from build123d import *

# Parameters (mm, degrees)
SKETCH1_W           = 30
SKETCH1_H           = 100
BOSS_EXTRUDE1_DEPTH = 5
SKETCH2_W           = 30
SKETCH2_H           = 45
BOSS_EXTRUDE2_DEPTH = 5
SKETCH3_W           = 30
SKETCH3_H           = 5
BOSS_EXTRUDE3_DEPTH = 15
SKETCH4_R           = 2.5
CUT_EXTRUDE1_DEPTH  = 8
SKETCH5_W           = 6
SKETCH5_H           = 5
CUT_EXTRUDE2_DEPTH  = 20


with BuildPart() as part:
    # Sketch1 → Boss-Extrude1 (new body)
    with BuildSketch(Plane.XY):
        with Locations((11.532089338, -8.646905221)):
            Rectangle(SKETCH1_W, SKETCH1_H)
        with BuildLine():
            Line((14.615865264, 31.346811585), (14.448313411, -48.653188415))
            ThreePointArc((14.448313411, -48.653188415), (11.442030217, -51.646905221), (8.448313411, -48.640622026))
            Line((8.448313411, -48.640622026), (8.615865264, 31.359377974))
            ThreePointArc((8.615865264, 31.359377974), (11.622148459, 34.353094779), (14.615865264, 31.346811585))
        make_face(mode=Mode.SUBTRACT)
    extrude(amount=BOSS_EXTRUDE1_DEPTH)

    # Sketch2 → Boss-Extrude2 (add)
    with BuildSketch(Plane(origin=(0, 41.353094779, 0), x_dir=(1, 0, 0), z_dir=(0, 1, 0))):
        with Locations((11.532089338, -2.5)):
            Rectangle(SKETCH2_W, SKETCH2_H)
    extrude(amount=BOSS_EXTRUDE2_DEPTH)

    # Sketch3 → Boss-Extrude3 (add)
    with BuildSketch(Plane(origin=(0, 46.353094779, 0), x_dir=(1, 0, 0), z_dir=(0, 1, 0))):
        with Locations((11.532089338, -2.5)):
            Rectangle(SKETCH3_W, SKETCH3_H)
    extrude(amount=BOSS_EXTRUDE3_DEPTH)

    # Sketch4 → Cut-Extrude1 (cut)
    with BuildSketch(Plane.XY.offset(5)):
        with Locations((21.532089338, 51.353094779)):
            Circle(SKETCH4_R)
    extrude(amount=-CUT_EXTRUDE1_DEPTH, mode=Mode.SUBTRACT)

    # Sketch5 → Cut-Extrude2 (cut)
    with BuildSketch(Plane(origin=(26.532089338, 0, 0), x_dir=(0, 0, -1), z_dir=(1, 0, 0))):
        with Locations((-8, 43.853094779)):
            Rectangle(SKETCH5_W, SKETCH5_H)
    extrude(amount=-CUT_EXTRUDE2_DEPTH, mode=Mode.SUBTRACT)


solid = part.part
The listing builds one solid part. Answer for the finished solid, in the listing's coordinates (mm). A direction names the side the tool comes from. Coordinates: 2 decimals unless noted, no trailing zeros. Write each loop counter-clockwise with the first axis right and the second up, starting at its lowest first coordinate (ties: lowest second). Pieces come first, ordered by that corner, then holes. Notation, with made-up numbers: M -35,-13.5 L -18,-13.5 A7 ccw -18,-0.5 Z; hole C 28,-17 d9. An arc over 180 degrees is marked long. Use one line per item in the form item = value.
Item 1: The mould has two halves that part along Y. Classify faces 5 (the face through (11, 41.353, -10)), 6 (the face through (26.532, 6, 1)), 7 (the face through (11.508, -51.646, 2.465)), 8 (the face through (11, 61.353, 2)): released by +Y, released by -Y, zero draft, split by the parting line, or undercut.
Model answer:
face_5 = released by -Y
face_6 = zero draft
face_7 = undercut
face_8 = released by +Y
Item 2: Find section B-B, the plane x = 1.5. Give the vertices of the cut face in (y, z).
Model answer:
outline = M -58.65,0 L 41.35,0 L 41.35,-20 L 46.35,-20 L 46.35,0 L 61.35,0 L 61.35,5 L 46.35,5 L 46.35,25 L 41.35,25 L 41.35,5 L -58.65,5 Z
Item 3: Find section C-C, the plane z = -5.5. Give the vertices of the cut face in (x, y), plus the area to 3 significant figures.
Model answer:
outline = M -3.47,41.35 L 26.53,41.35 L 26.53,46.35 L -3.47,46.35 Z
area = 150 mm2
Item 4: Find the intervals of material crossed by probe 1 along Z at (x, y) = (17.5, 42.5); probe 2 along Y at (x, z) = (14, 12.5); probe 3 along Z at (x, y) = (18.25, -26.5), in increasing order.
Model answer:
probe_1 = -20 to 5, 11 to 25
probe_2 = 41.35 to 46.35
probe_3 = 0 to 5
Item 5: Find section A-A, the plane y = 27.5. Give the vertices of the cut face in (x, z), plus the area to 3 significant figures.
Model answer:
outline = M -3.47,0 L 8.61,0 L 8.61,5 L -3.47,5 Z; M 14.61,0 L 26.53,0 L 26.53,5 L 14.61,5 Z
area = 120 mm2
Item 6: For faces 1 (the face through (11, 41.353, 17)), 2 (the face through (11, 54, 0)), 3 (the face through (17, 44, 11)), 4 (the face through (8, -8, 0)), determine the directions among +Z, -Z, +X, -X, +Y, -Y from which every point of the face is accessible in a straight line to the end or side of a thin tool.
Model answer:
face_1 = +Z, +X, -X, -Y
face_2 = -Z, +X, -X, +Y
face_3 = +X, +Y, -Y
face_4 = -Z, +X, -X, -Y
Item 7: Given P1, Ø5.5, axis at y = 45, z = 7, coming from the +X side; P2, Ø6, axis at x = 15.5, z = -5, coming from the +Y side; P3, Ø4, axis at x = 4.5, y = 20.5, coming from the +Z side; P4, Ø16, axis at x = 6.5, z = 19, coming from the -Y side, each flat-ended and moving along its own axis, determine where each tip first touches the part or whether it passes through.
Model answer:
P1 = 26.53
P2 = 46.35
P3 = 5
P4 = 41.35
